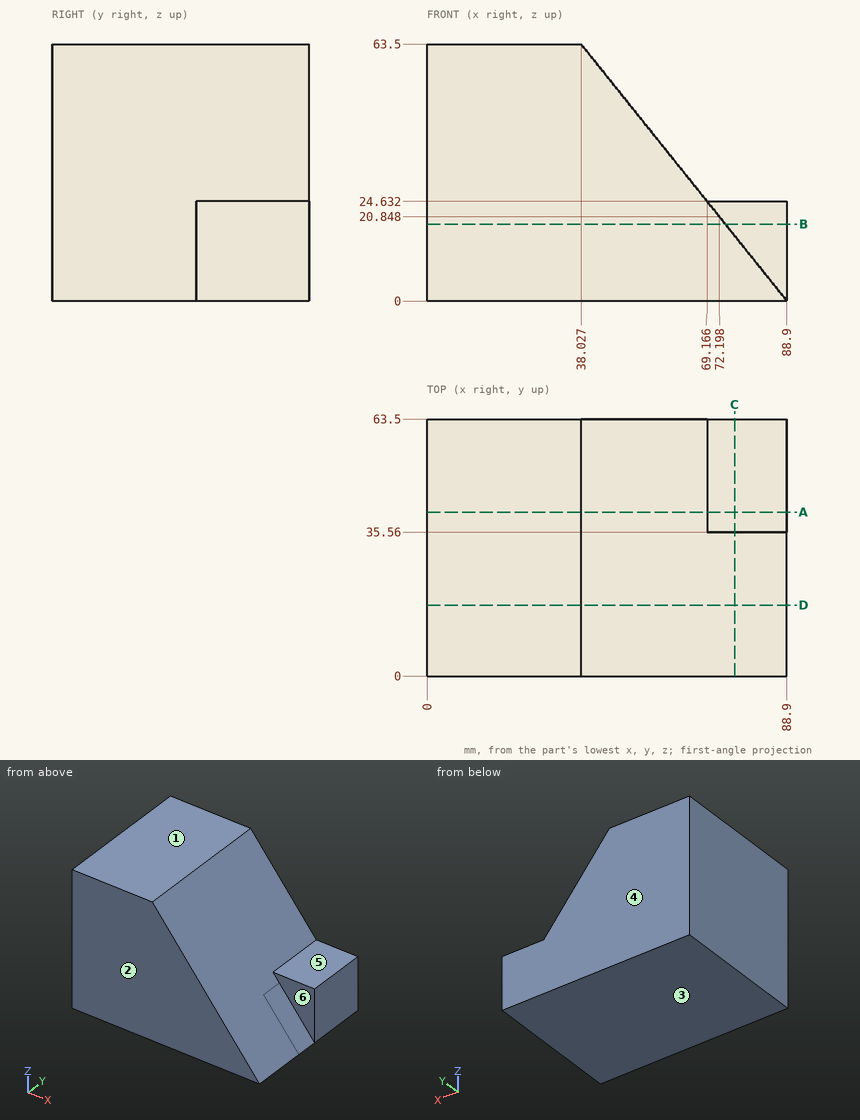
Here's the drawing with two shaded views (mm, measured from the low corner). I have some questions. A direction names the side the tool comes from. Coordinates: 2 decimals unless noted, no trailing zeros. Loops run counter-clockwise (first coordinate to the right, second up) from the corner with the lowest first, then second, coordinate; pieces in that order, holes last. Notation, with made-up numbers: (61.25, -21) -> (73.25, -21) arc R31 cw to (73.25, 12) -> close; hole circle Ø10 at (53.25, 83). An arc over 180 degrees is marked (long way). Use one line per item in the form item = value. Start each with the question number.
(1) On a 3-axis mill with a long thin cutter (end or side, diameter ignored), from which of +Z, -Z, +X, -X, +Y, -Y can I reach the whole of each face in a straight line? I mean the marked faces 4, 5 and 6. Say none if no direction works.
(2) If we section it at A-A (y = 40.5): Please give me the cut outline in (x, z), then the cut area to 3 significant figures.
(3) Please list where these lines run through material, in increasing order: line 1 along Y through (x, z) = (83, 19); line 2 along X through (y, z) = (17, 55); line 3 along Z through (x, y) = (46.5, 56.5) (1 decimal).
(4) If we section it at C-C (x = 76): Please give me the cut outline in (y, z).
(5) We'd pull the mould along Z, two halves only. Please class the marked faces 1, 2 and 3: pulls with the +Z half, pulls with the -Z half, needs draft (parallel to the pull), parting line crosses it, or undercut.
(6) If we section it at B-B (z = 19): Please give me the cut outline in (x, y), then the cut area to 3 significant figures.
(7) Will these pins go through, and if not, where does the flat tip stop? pin 1 (3 mm diameter, centred on x = 67, y = 39, fed in from +Z); pin 2 (21.5 mm diameter, centred on x = 76, y = 46.5, fed in from +Z).
(8) If we section it at D-D (y = 17.5): Please give me the cut outline in (x, z), then the cut area to 3 significant figures.
Verdict:
q1.face_4 = +Z, -Z, +X, -X, +Y
q1.face_5 = +Z, +X, +Y, -Y
q1.face_6 = +Z, +X, -Y
q2.outline = (0, 0) -> (88.9, 0) -> (88.9, 24.63) -> (69.17, 24.63) -> (38.03, 63.5) -> (0, 63.5) -> close
q2.area = 4,270 mm²
q3.line_1 = 35.56 to 63.5
q3.line_2 = 0 to 44.84
q3.line_3 = 0 to 52.9
q4.outline = (0, 0) -> (63.5, 0) -> (63.5, 24.63) -> (35.56, 24.63) -> (35.56, 16.1) -> (0, 16.1) -> close
q5.face_1 = pulls with the +Z half
q5.face_2 = needs draft
q5.face_3 = pulls with the -Z half
q6.outline = (0, 0) -> (73.68, 0) -> (73.68, 35.56) -> (88.9, 35.56) -> (88.9, 63.5) -> (0, 63.5) -> close
q6.area = 5,100 mm²
q7.pin_1 = 29.21
q7.pin_2 = 29.52
q8.outline = (0, 0) -> (88.9, 0) -> (38.03, 63.5) -> (0, 63.5) -> close
q8.area = 4,030 mm²
